```python
from build123d import *

# Parameters (mm, degrees)
EXTRUDE1_DEPTH       = 8.382
SKETCH2_R            = 3.96875
CUT_EXTRUDE1_DEPTH   = 172.593904288
FILLET4_R            = 9.525
FILLET4_OF_MIRROR1_R = 9.525


with BuildPart() as part:
    # Sketch1 → Extrude1 (new body)
    with BuildSketch(Plane.XY):
        Polygon((0, 0), (0, 29.903849897), (46.305765967, 156.371903759), (70.157236117, 147.638784517), (25.4, 25.4), (25.4, 0), align=None)
    extrude1 = extrude(amount=EXTRUDE1_DEPTH)

    # Sketch2 → Cut-Extrude1 (cut, through all)
    with BuildSketch(Plane(origin=(0, 0, 0), x_dir=(-1, 0, 0), z_dir=(0, 0, -1))):
        with Locations((-53.864941421, 140.079609063)):
            Circle(SKETCH2_R)
        with Locations((-12.7, 15.875)):
            Circle(SKETCH2_R)
    cut_extrude1 = extrude(amount=-CUT_EXTRUDE1_DEPTH, mode=Mode.SUBTRACT)

    # Fillet4
    fillet4_edges = [part.edges().sort_by_distance(p)[0] for p in [
        (46.305765967, 156.371903759, 4.191),
        (70.157236117, 147.638784517, 4.191),
    ]]
    fillet(fillet4_edges, radius=FILLET4_R)

    # Mirror1: Extrude1, Cut-Extrude1 across plane
    add(extrude1.mirror(Plane(origin=(25.4, 0, 8.382), x_dir=(0, 0, 1), z_dir=(0, 1, 0))))
    add(cut_extrude1.mirror(Plane(origin=(25.4, 0, 8.382), x_dir=(0, 0, 1), z_dir=(0, 1, 0))), mode=Mode.SUBTRACT)

    # Fillet4 of Mirror1
    fillet4_of_mirror1_edges = [part.edges().sort_by_distance(p)[0] for p in [
        (46.305765967, -156.371903759, 4.191),
        (70.157236117, -147.638784517, 4.191),
    ]]
    fillet(fillet4_of_mirror1_edges, radius=FILLET4_OF_MIRROR1_R)


solid = part.part
```
Geometry check sheet. Reference: the model listing, model coordinates, mm. A direction names the side the tool comes from. Round coordinates to 2 decimals unless told otherwise and drop trailing zeros. Loops run counter-clockwise (first coordinate to the right, second up) from the corner with the lowest first, then second, coordinate; pieces in that order, holes last. Notation, with made-up numbers: (45, 70) - (95, 70) arc R22 cw to (95, 87) - close; hole circle Ø8 at (61, 59.5). An arc over 180 degrees is marked (long way). Use a Markdown table: item, result.
Q1. Draft check along Y on faces 3 (the flat face through (19, -2, 8.382)), 4 (the flat face through (46.43, 82.84, 4.13)), 5 (the flat face through (58.19, 152.02, 4.13)), 6 (the flat face through (46.43, -82.84, 4.13)). Enter one of: released by +Y, released by -Y, zero draft, split by the parting line, or undercut.
Solutions:
| item | result |
|---|---|
| face 3 | zero draft |
| face 4 | undercut |
| face 5 | released by +Y |
| face 6 | undercut |
Q2. Cross-section at C-C on z = 2.5. State how many separate pieces and enclosed holes the cut face has, plus the area to 3 significant figures.
Solutions:
| item | result |
|---|---|
| separate pieces | 1 |
| enclosed holes | 4 |
| area | 7,860 mm2 |
Q3. Access from +Z, -Z, +X, -X, +Y, -Y to the whole of each face (thin tool, end or side, straight path). Record for faces 1 (the flat face through (58.19, -152.02, 4.13)), 2 (the flat face through (25.4, 0, 4)).
Solutions:
| item | result |
|---|---|
| face 1 | +Z, -Z, +X, -Y |
| face 2 | +Z, -Z, +X |
Q4. Cross-section at A-A on x = 12.7. Record the cut outline in (y, z).
Solutions:
| item | result |
|---|---|
| outline | (-64.59, 0) - (-19.84, 0) - (-19.84, 8.38) - (-64.59, 8.38) - close; (-11.91, 0) - (11.91, 0) - (11.91, 8.38) - (-11.91, 8.38) - close; (19.84, 0) - (64.59, 0) - (64.59, 8.38) - (19.84, 8.38) - close |
Q5. Go/stop test with flat-tipped pins: P1, Ø6.5, axis at x = 53.86, y = -140.08, coming from the +Z side; P2, Ø2, axis at y = 47.5, z = 4, coming from the -X side. Record where each tip stops, or that it passes through.
Solutions:
| item | result |
|---|---|
| P1 | passes through |
| P2 | stops at x = 6.08 |
Q6. Cross-section at D-D on y = -50. Record the cut outline in (x, z), plus the area to 3 significant figures.
Solutions:
| item | result |
|---|---|
| outline | (7.36, 0) - (34.41, 0) - (34.41, 8.38) - (7.36, 8.38) - close |
| area | 227 mm2 |
Q7. Cross-section at B-B on x = 46.5. Record the cut outline in (y, z), plus the area to 3 significant figures.
Solutions:
| item | result |
|---|---|
| outline | (-151.95, 0) - (-83.03, 0) - (-83.03, 8.38) - (-151.95, 8.38) - close; (83.03, 0) - (151.95, 0) - (151.95, 8.38) - (83.03, 8.38) - close |
| area | 1,160 mm2 |
Q8. Material ranges on line 1 (X direction, y = -4, z = 6); line 2 (X direction, y = 19.5, z = 2.75); line 3 (X direction, y = 38, z = 6.25), recorded low to high.
Solutions:
| item | result |
|---|---|
| line 1 | x = 0 to 25.4 |
| line 2 | x = 0 to 11.08, 14.32 to 25.4 |
| line 3 | x = 2.96 to 30.01 |
